```python
from build123d import *

# Parameters (mm, degrees)
F3_DEPTH = 50
F4_DEPTH = 50
F5_DEPTH = 50


with BuildPart() as f3:
    # F0 (on Top) → F3 (new body, symmetric)
    with BuildSketch(Plane.XY):
        Polygon((15, 50), (0, 50), (-15, 50), (-50, -50), (-26.013944, -50), (-17.136321, -20), (17.136321, -20), (26.013944, -50), (50, -50), align=None)
        Polygon((-11.217906, 0), (0, 37.90848), (11.217906, 0), align=None, mode=Mode.SUBTRACT)
    extrude(amount=F3_DEPTH, both=True)

    # F1 (on Front) → F4 (intersect, symmetric)
    with BuildSketch(Plane.XZ):
        with BuildLine():
            Line((50, 30.683344), (50, 50))
            Line((50, 50), (-34.83974, 50))
            Line((-34.83974, 50), (-34.83974, 30.683344))
            Line((-34.83974, 30.683344), (-6.906417, 30.683344))
            Line((-6.906417, 30.683344), (-6.906417, -20.520055))
            ThreePointArc((-6.906417, -20.520055), (-8.370883, -24.055589), (-11.906417, -25.520055))
            Line((-11.906417, -25.520055), (-14.371657, -25.520055))
            ThreePointArc((-14.371657, -25.520055), (-17.907191, -24.055589), (-19.371657, -20.520055))
            Line((-19.371657, -20.520055), (-19.371657, -9.06684))
            Line((-19.371657, -9.06684), (-50, -9.06684))
            Line((-50, -9.06684), (-50, -45))
            ThreePointArc((-50, -45), (-48.535534, -48.535534), (-45, -50))
            Line((-45, -50), (17.066677, -50))
            ThreePointArc((17.066677, -50), (20.602211, -48.535534), (22.066677, -45))
            Line((22.066677, -45), (22.066677, 30.683344))
            Line((22.066677, 30.683344), (50, 30.683344))
        make_face()
    extrude(amount=F4_DEPTH, both=True, mode=Mode.INTERSECT)

    # F2 (on Right) → F5 (intersect, symmetric)
    with BuildSketch(Plane.YZ):
        with BuildLine():
            Line((18.11799, 17.495545), (35.967778, 34.732102))
            ThreePointArc((35.967778, 34.732102), (-50, 0), (35.967778, -34.732102))
            Line((35.967778, -34.732102), (18.11799, -17.495545))
            ThreePointArc((18.11799, -17.495545), (-25.186418, 0), (18.11799, 17.495545))
        make_face()
    extrude(amount=F5_DEPTH, both=True, mode=Mode.INTERSECT)


solid = f3.part
```
Could you check a few things on this model? Use its own coordinates, in mm. A direction names the side the tool comes from. Round coordinates to 2 decimals unless told otherwise and drop trailing zeros. Loops run counter-clockwise (first coordinate to the right, second up) from the corner with the lowest first, then second, coordinate; pieces in that order, holes last. Notation, with made-up numbers: (84.5, 23) -> (138.5, 23) arc R18 cw to (138.5, 50) -> close; hole circle Ø9 at (2.25, 31.25). An arc over 180 degrees is marked (long way). Put each result on its own line as item: value.
Q1. Thinking about a two-plate mould opening in Z: for faces 5 (the flat face through (-29, 10, 38)), 6 (the cylindrical face through (-13.319, -3.23, -49.896)), 7 (the flat face through (-6.906, 21, 26)), 8 (the flat face through (-19.372, -23, -16)), which applies, pulls with the +Z half, pulls with the -Z half, needs draft (parallel to the pull), parting line crosses it, or undercut?
Checks:
face 5: needs draft
face 6: pulls with the -Z half
face 7: undercut
face 8: undercut
Q2. I want a section at B-B on z = 0. Write out the boundary of the cut face in (x, y), and give its area (3 significant figures).
Checks:
outline: (18.67, -25.19) -> (22.07, -36.66) -> (22.07, -25.19) -> close
area: 19.5 mm2
Q3. Which directions (+Z, -Z, +X, -X, +Y, -Y) give clear straight access to the entire face, cutting with the end or side of a thin tool? Please do faces 1 (the cylindrical face through (-25.55, -10.01, -23.11)), 2 (the flat face through (-21, -4, 30.683)), 3 (the flat face through (-20.554, -31.548, -23.105)), 4 (the flat face through (-6.906, -19, -19)).
Checks:
face 1: +X, -X
face 2: -X, +Y, -Y
face 3: +Z, -Z, -Y
face 4: +Y, -Y
Q4. Please list where these lines run through material, in increasing order: line 1 (Z direction, x = 11.5, y = 0); line 2 (Y direction, x = 14, z = -18); line 3 (Z direction, x = 8, y = -11) (3 decimals). Write a range as from..to.
Checks:
line 1: -50..-25.19, 25.19..50
line 2: -20..-17.62, 17.62..18.64
line 3: -48.775..-22.657, 22.657..48.775
Q5. For pin 1 Ø6 at (x, y) = (-30.5, 6) entering from -Z; pin 2 Ø1 at (x, y) = (31, -7.5) entering from -Z; pin 3 Ø1.5 at (y, z) = (18, -18.5) entering from -X, each with a flat end and sliding along its axis, tell me the tip position at first contact or that it passes through.
Checks:
pin 1: z = -49.91
pin 2: z = 30.68
pin 3: x = -26.46
Q6. I want a section at A-A on x = 29.5. Write out the boundary of the cut face in (y, z).
Checks:
outline: (-39.48, 30.68) -> (8.57, 30.68) -> (8.57, 49.26) arc R50 ccw to start
